from build123d import *

# Parameters (mm, degrees)
F1_DEPTH = 63.5
F0_W     = 28.575
F0_H     = 19.05
F2_DEPTH = 25.4
F3_DEPTH = 7.9375
F5_R     = 6.35
F6_R     = 5.08
F7_DEPTH = 25.4
F8_R     = 19.05
F9_DEPTH = 36.83


with BuildPart() as f1:
    # F0 (on Front) → F1 (new body, symmetric)
    with BuildSketch(Plane.XZ):
        Polygon((41.275, -9.525), (41.275, 9.525), (22.225, 9.525), (-41.275, 9.525), (-41.275, -9.525), align=None)
    extrude(amount=F1_DEPTH, both=True)

    # F0 (on Front) → F2 (join, symmetric)
    with BuildSketch(Plane.XZ):
        with BuildLine():
            Line((22.225, 9.525), (41.275, 9.525))
            Line((41.275, 9.525), (41.275, 27.0002))
            ThreePointArc((41.275, 27.0002), (45.92468, 38.22552), (57.15, 42.8752))
            Line((57.15, 42.8752), (57.15, 61.9252))
            ThreePointArc((57.15, 61.9252), (32.454296, 51.695904), (22.225, 27.0002))
            Line((22.225, 27.0002), (22.225, 9.525))
        make_face()
        with Locations((71.4375, 52.4002)):
            Rectangle(F0_W, F0_H)
    extrude(amount=F2_DEPTH, both=True)

    # F0 (on Front) → F3 (join, symmetric)
    with BuildSketch(Plane.XZ):
        with BuildLine():
            Line((-41.275, 9.525), (22.225, 9.525))
            Line((22.225, 9.525), (22.225, 27.0002))
            ThreePointArc((22.225, 27.0002), (32.454296, 51.695904), (57.15, 61.9252))
            add(Edge.make_bspline(
                [(-41.275, 9.525), (-38.595248, 38.531583), (15.192084, 62.063541), (57.15, 61.9252)],
                knots=[0, 0, 0, 0, 111.504536, 111.504536, 111.504536, 111.504536], degree=3))
        make_face()
    extrude(amount=F3_DEPTH, both=True)

    # F0 (on Front) → F4 (revolve)
    with BuildSketch(Plane.XZ):
        Polygon((85.725, 61.9252), (85.725, 42.8752), (85.725, 36.837653), (114.3, 36.837653), (114.3, 66.675), (85.725, 66.675), align=None)
    revolve(axis=Axis((85.725, 0, 52.4002), (0, 0, -1)))

    # F5
    f5_edges = [f1.edges().sort_by_distance(p)[0] for p in [
        (-41.275, -63.5, 0),
        (41.275, -63.5, 0),
        (-41.275, 63.5, 0),
        (41.275, 63.5, 0),
    ]]
    fillet(f5_edges, radius=F5_R)

    # F6 (on face) → F7 (cut)
    with BuildSketch(Plane.XY.offset(9.525)):
        with Locations((-31.115, 53.34)):
            Circle(F6_R)
        with Locations((31.115, 53.34)):
            Circle(F6_R)
        with Locations((-31.115, -53.34)):
            Circle(F6_R)
        with Locations((31.115, -53.34)):
            Circle(F6_R)
    extrude(amount=-F7_DEPTH, mode=Mode.SUBTRACT)

    # F8 (on face) → F9 (cut)
    with BuildSketch(Plane.XY.offset(66.675)):
        with Locations((85.725, 0)):
            Circle(F8_R)
    extrude(amount=-F9_DEPTH, mode=Mode.SUBTRACT)


solid = f1.part
Design review of the part built by this model. Coordinates are the model's own, in mm. A direction names the side the tool comes from. Give positions to 0.01 mm unless a question says otherwise; leave off trailing zeros. Loops run counter-clockwise (first coordinate to the right, second up) from the corner with the lowest first, then second, coordinate; pieces in that order, holes last. Notation, with made-up numbers: M -4.5,62 L 24.5,62 A5 cw 24.5,71 Z; hole C -28.75,78 d4. An arc over 180 degrees is marked long. One line per question, with ' | ' between items. Start each with the question number.
1. For faces 1 (the face through (61, -18, 42.875)), 2 (the face through (22.225, 17, 18)), 3 (the face through (-4, -7.938, 30)), list the 3-axis set-ups (+Z, -Z, +X, -X, +Y, -Y) from which the entire face can be reached by the end or side of a thin tool; tool diameter is ignored.
2. Add section C-C (y = -16). Write out the cut boundary in (x, z) (3 decimals).
3. Insertion check: P1, Ø3, axis at x = -13.5, y = -36, coming from the +Z side (3 decimals); P2, Ø17, axis at x = 87.5, y = -3.5, coming from the -Z side; P3, Ø17, axis at x = 63.5, y = -12, coming from the -Z side; P4, Ø8.5, axis at y = 17, z = 22.5, coming from the -X side (3 decimals). Each pin has a flat end and moves straight along its axis. Give the tip position at first contact, or say it passes through.
4. The part is to be moulded in two halves that separate along Y. For faces 4 (the face through (39.464, -61.59, 0.133)), 5 (the face through (80, 19, 36.838)), 6 (the face through (27.084, -56.431, 0.133)), say which applies: released by +Y, released by -Y, zero draft, split by the parting line, or undercut.
5. Add section A-A (y = 53.34). Write out the cut boundary in (x, z) (3 decimals).
6. To check wall thickness, follow L1, parallel to X at y = 53, z = -1 (3 decimals); L2, parallel to Y at x = 86.5, z = 43; L3, parallel to Y at x = 45, z = 55.5. State the ranges of each line that lie inside material, in increasing order.
7. Add section D-D (y = -34.5). Write out the cut boundary in (x, z) (3 decimals).
8. Add section B-B (x = 86). Write out the cut boundary in (y, z) (3 decimals).
Worked out:
1) face 1: -Z, -Y | face 2: +Z, -X, +Y | face 3: +Z, -X, -Y
2) outline: M -41.275,-9.525 L 41.275,-9.525 L 41.275,27 A15.875 cw 57.15,42.875 L 62.049,42.875 L 62.049,36.838 L 75.386,36.838 L 75.386,66.675 L 62.049,66.675 L 62.049,61.925 L 57.15,61.925 A34.925 ccw 22.225,27 L 22.225,9.525 L -41.275,9.525 Z; M 96.064,36.838 L 109.401,36.838 L 109.401,66.675 L 96.064,66.675 Z
3) P1: stops at z = 9.525 | P2: passes through | P3: stops at z = 36.84 | P4: stops at x = 22.225
4) face 4: released by -Y | face 5: zero draft | face 6: undercut
5) outline: M -41.275,-9.525 L -36.195,-9.525 L -36.195,9.525 L -41.275,9.525 Z; M -26.035,-9.525 L 26.035,-9.525 L 26.035,9.525 L -26.035,9.525 Z; M 36.195,-9.525 L 41.275,-9.525 L 41.275,9.525 L 36.195,9.525 Z
6) L1: x = -41.275 to -36.184, -26.046 to 26.046, 36.184 to 41.275 | L2: y = -28.56 to -19.03, 19.03 to 28.56 | L3: y = -25.4 to 25.4
7) outline: M -41.275,-9.525 L 41.275,-9.525 L 41.275,9.525 L -41.275,9.525 Z
8) outline: M -28.574,36.838 L -19.048,36.838 L -19.048,66.675 L -28.574,66.675 Z; M 19.048,36.838 L 28.574,36.838 L 28.574,66.675 L 19.048,66.675 Z
